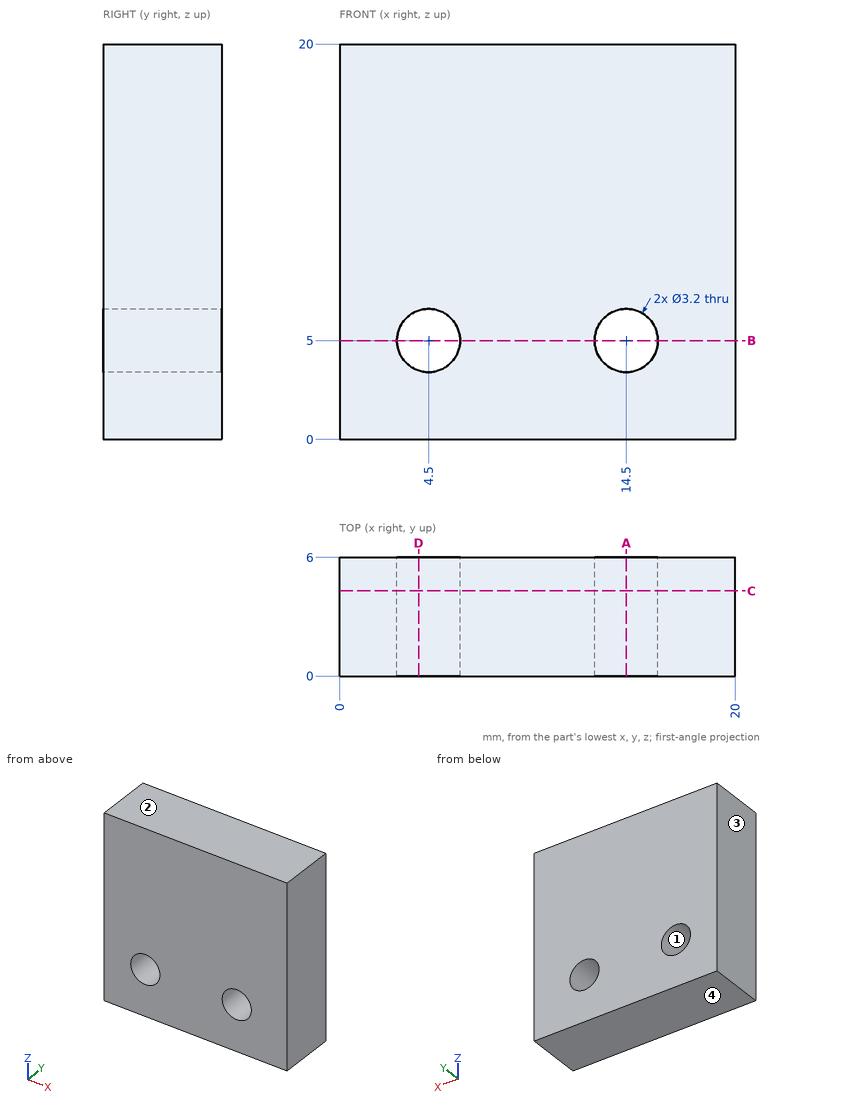
Geometry: see drawing. Coordinates: mm, zero at the bounding-box minimum. Coordinates: 2 decimals unless noted, no trailing zeros. Loops run counter-clockwise (first coordinate to the right, second up) from the corner with the lowest first, then second, coordinate; pieces in that order, holes last.
(1) Section C-C on y = 4.3. Return the cut outline in (x, z).
(2) Section D-D on x = 4. Return the cut outline in (y, z), then the cut area to 3 significant figures.
(3) Section A-A on x = 14.5. Return the cut outline in (y, z).
(4) Section B-B on z = 5. Return the cut outline in (x, y), then the cut area to 3 significant figures.
(5) Material intervals for probe 1 along X at (y, z) = (4.75, 5); probe 2 along Z at (x, y) = (14.5, 1.65); probe 3 along X at (y, z) = (5.25, 4.25), sorted ascending.
(6) Pull-direction query (Z, two-part tool) for the marked faces 1, 2, 3 and 4; classes: released by +Z, released by -Z, zero draft, split by the parting line, or undercut.
Data:
1. outline: (0, 0) - (20, 0) - (20, 20) - (0, 20) - close; hole circle Ø3.2 at (4.5, 5); hole circle Ø3.2 at (14.5, 5)
2. outline: (0, 0) - (6, 0) - (6, 3.48) - (0, 3.48) - close; (0, 6.52) - (6, 6.52) - (6, 20) - (0, 20) - close
2. area: 102 mm2
3. outline: (0, 0) - (6, 0) - (6, 3.4) - (0, 3.4) - close; (0, 6.6) - (6, 6.6) - (6, 20) - (0, 20) - close
4. outline: (0, 0) - (2.9, 0) - (2.9, 6) - (0, 6) - close; (6.1, 0) - (12.9, 0) - (12.9, 6) - (6.1, 6) - close; (16.1, 0) - (20, 0) - (20, 6) - (16.1, 6) - close
4. area: 81.6 mm2
5. probe 1: x = 0 to 2.9, 6.1 to 12.9, 16.1 to 20
5. probe 2: z = 0 to 3.4, 6.6 to 20
5. probe 3: x = 0 to 3.09, 5.91 to 13.09, 15.91 to 20
6. face 1: undercut
6. face 2: released by +Z
6. face 3: zero draft
6. face 4: released by -Z
